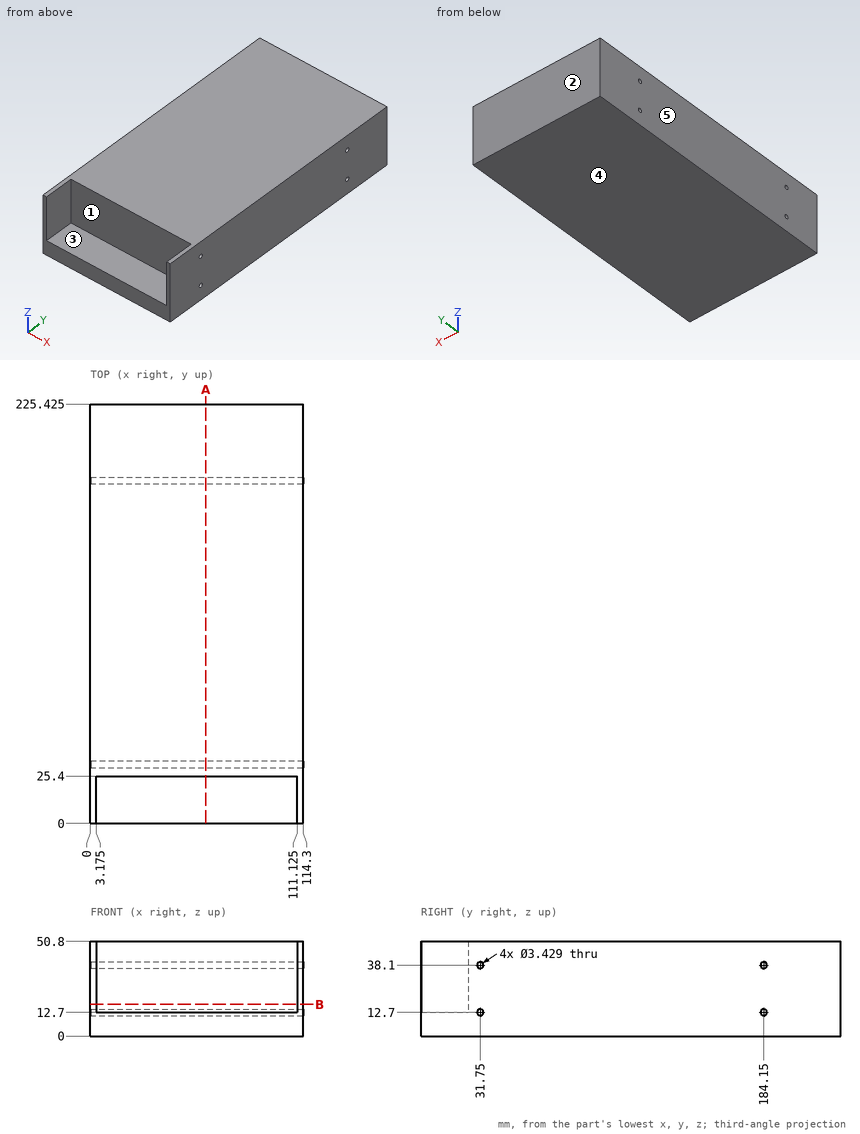
Design review of the part shown in the three views and the two pictorial views. Dimensions are in mm from the part's minimum x, y and z. A direction names the side the tool comes from. Coordinates: 2 decimals unless noted, no trailing zeros. Write each loop counter-clockwise with the first axis right and the second up, starting at its lowest first coordinate (ties: lowest second). Pieces come first, ordered by that corner, then holes.
1) We need section B-B on z = 17. State the section outline as (x, y) points (3 decimals), then the cut area to 3 significant figures.
2) To check wall thickness, follow probe 1 along Y at (x, z) = (70, 38) (3 decimals); probe 2 along Z at (x, y) = (37, 31.75); probe 3 along Z at (x, y) = (47, 31). State the ranges of each line that lie inside material, in increasing order.
3) We need section A-A on x = 62. Count the separate pieces of the cut face and the enclosed holes in it, then the cut area to 3 significant figures.
4) Clearance check with flat-ended pins moving along their axes: pin 1 Ø4 at (y, z) = (31.75, 12.7) entering from -X; pin 2 Ø1.5 at (x, z) = (54.5, 15) entering from -Y; pin 3 Ø12.5 at (x, y) = (47.5, 11) entering from +Z. State where each tip first meets the part, or that it passes through.
5) Machinability: for the marked faces 1 and 2, which of the approach directions +Z, -Z, +X, -X, +Y, -Y give a long, thin tool a straight path to every point of the face, cutting with its end or side? Answer none if there is none.
6) The part is to be moulded in two halves that separate along X. For the marked faces 3, 4 and 5, say which applies: pulls with the +X half, pulls with the -X half, needs draft (parallel to the pull), parting line crosses it, or undercut.
Answer list:
1. outline: (0, 0) - (3.175, 0) - (3.175, 25.4) - (111.125, 25.4) - (111.125, 0) - (114.3, 0) - (114.3, 225.425) - (0, 225.425) - close
1. area: 23,000 mm2
2. probe 1: y = 25.4 to 30.038, 33.462 to 182.438, 185.862 to 225.425
2. probe 2: z = 0 to 10.99, 14.41 to 36.39, 39.81 to 50.8
2. probe 3: z = 0 to 11.16, 14.24 to 36.56, 39.64 to 50.8
3. separate pieces: 1
3. enclosed holes: 4
3. area: 10,400 mm2
4. pin 1: stops at x = 0
4. pin 2: stops at y = 25.4
4. pin 3: stops at z = 12.7
5. face 1: +Z, -Y
5. face 2: +Z, -Z, +X, -X, +Y
6. face 3: undercut
6. face 4: needs draft
6. face 5: pulls with the -X half
